Source: CAD feature listing. Evaluate the final solid. Frame: model axes, mm. Coordinates: 2 decimals unless noted, no trailing zeros. Order: outer loops, then holes, each group sorted by start corner. A loop starts at its lowest first (then second) coordinate and runs counter-clockwise, first axis right, second up. Notation, with made-up numbers: (81.25, 55) -> (135.25, 55) arc R21 cw to (135.25, 76) -> close; hole circle Ø5 at (38, 66). An arc over 180 degrees is marked (long way). Write item = value, one per line. Start each with the question number.
Item 1: Ray query, line 1 along X through (y, z) = (5, -38); line 2 along X through (y, z) = (14.25, 42); line 3 along Z through (x, y) = (210.5, 2.75). Return the intervals inside material, ascending. Write a range as [from, to].
Item 2: Contact query for flat-ended pins moving along their axis: pin 1 (1 mm diameter, centred on x = -160.5, z = 70.5, fed in from -Y); pin 2 (5 mm diameter, centred on y = 2.5, z = 75.5, fed in from -X). Output: stop coordinate, or through.
Item 3: Section query A-A (z = 84.5). Output: boundary loops of the cut face in (x, y), then the cut area to 3 significant figures.
```python
from build123d import *

# Parameters (mm, degrees)
BOSS_EXTRUDE1_DEPTH = 15
CUT_EXTRUDE2_DEPTH  = 16
SKETCH4_W           = 524.5681158
SKETCH4_H           = 94.971164408
CUT_EXTRUDE3_DEPTH  = 30


with BuildPart() as part:
    # Sketch1 → Boss-Extrude1 (new body)
    with BuildSketch(Plane(origin=(0, 0, 0), x_dir=(1, 0, 0), z_dir=(0, 1, 0))):
        with BuildLine():
            Line((-200, -100), (200, -100))
            ThreePointArc((200, -100), (221.213203436, -91.213203436), (230, -70))
            Line((230, -70), (230, 100))
            Line((230, 100), (-230, 100))
            Line((-230, 100), (-230, -70))
            ThreePointArc((-230, -70), (-221.213203436, -91.213203436), (-200, -100))
        make_face()
    extrude(amount=BOSS_EXTRUDE1_DEPTH)

    # Sketch3 → Cut-Extrude2 (cut, through all)
    with BuildSketch(Plane(origin=(0, 15, 0), x_dir=(1, 0, 0), z_dir=(0, 1, 0))):
        with BuildLine():
            Line((-2466.524123707, -5837.229065469), (-2474.461623707, -5841.991565469))
            ThreePointArc((-2474.461623707, -5841.991565469), (-2480.995719801, -5840.358041446), (-2479.362195777, -5833.823945352))
            Line((-2479.362195777, -5833.823945352), (-2471.424695777, -5829.061445352))
            ThreePointArc((-2471.424695777, -5829.061445352), (-2464.890599684, -5830.694969376), (-2466.524123707, -5837.229065469))
        make_face()
        with BuildLine():
            Line((-2466.524123707, -5905.261445352), (-2474.461623707, -5900.498945352))
            ThreePointArc((-2474.461623707, -5900.498945352), (-2480.995719801, -5902.132469376), (-2479.362195777, -5908.666565469))
            Line((-2479.362195777, -5908.666565469), (-2471.424695777, -5913.429065469))
            ThreePointArc((-2471.424695777, -5913.429065469), (-2464.890599684, -5911.795541446), (-2466.524123707, -5905.261445352))
        make_face()
        with BuildLine():
            Line((-2395.224695777, -5837.229065469), (-2387.287195777, -5841.991565469))
            ThreePointArc((-2387.287195777, -5841.991565469), (-2380.753099684, -5840.358041446), (-2382.386623707, -5833.823945352))
            Line((-2382.386623707, -5833.823945352), (-2390.324123707, -5829.061445352))
            ThreePointArc((-2390.324123707, -5829.061445352), (-2396.858219801, -5830.694969376), (-2395.224695777, -5837.229065469))
        make_face()
        with BuildLine():
            Line((-2395.224695777, -5905.261445352), (-2387.287195777, -5900.498945352))
            ThreePointArc((-2387.287195777, -5900.498945352), (-2380.753099684, -5902.132469376), (-2382.386623707, -5908.666565469))
            Line((-2382.386623707, -5908.666565469), (-2390.324123707, -5913.429065469))
            ThreePointArc((-2390.324123707, -5913.429065469), (-2396.858219801, -5911.795541446), (-2395.224695777, -5905.261445352))
        make_face()
        with BuildLine():
            Line((-34.016189941, -35.649713965), (-29.253689941, -43.587213965))
            ThreePointArc((-29.253689941, -43.587213965), (-30.887213965, -50.121310059), (-37.421310059, -48.487786035))
            Line((-37.421310059, -48.487786035), (-42.183810059, -40.550286035))
            ThreePointArc((-42.183810059, -40.550286035), (-40.550286035, -34.016189941), (-34.016189941, -35.649713965))
        make_face()
        with BuildLine():
            Line((34.016189941, -35.649713965), (29.253689941, -43.587213965))
            ThreePointArc((29.253689941, -43.587213965), (30.887213965, -50.121310059), (37.421310059, -48.487786035))
            Line((37.421310059, -48.487786035), (42.183810059, -40.550286035))
            ThreePointArc((42.183810059, -40.550286035), (40.550286035, -34.016189941), (34.016189941, -35.649713965))
        make_face()
        with BuildLine():
            Line((-34.016189941, 35.649713965), (-29.253689941, 43.587213965))
            ThreePointArc((-29.253689941, 43.587213965), (-30.887213965, 50.121310059), (-37.421310059, 48.487786035))
            Line((-37.421310059, 48.487786035), (-42.183810059, 40.550286035))
            ThreePointArc((-42.183810059, 40.550286035), (-40.550286035, 34.016189941), (-34.016189941, 35.649713965))
        make_face()
        with BuildLine():
            Line((34.016189941, 35.649713965), (29.253689941, 43.587213965))
            ThreePointArc((29.253689941, 43.587213965), (30.887213965, 50.121310059), (37.421310059, 48.487786035))
            Line((37.421310059, 48.487786035), (42.183810059, 40.550286035))
            ThreePointArc((42.183810059, 40.550286035), (40.550286035, 34.016189941), (34.016189941, 35.649713965))
        make_face()
    extrude(amount=-CUT_EXTRUDE2_DEPTH, mode=Mode.SUBTRACT)

    # Sketch4 → Cut-Extrude3 (cut)
    with BuildSketch(Plane(origin=(0, 0, -100), x_dir=(-1, 0, 0), z_dir=(0, 0, -1))):
        Rectangle(SKETCH4_W, SKETCH4_H)
    extrude(amount=-CUT_EXTRUDE3_DEPTH, mode=Mode.SUBTRACT)


solid = part.part
```
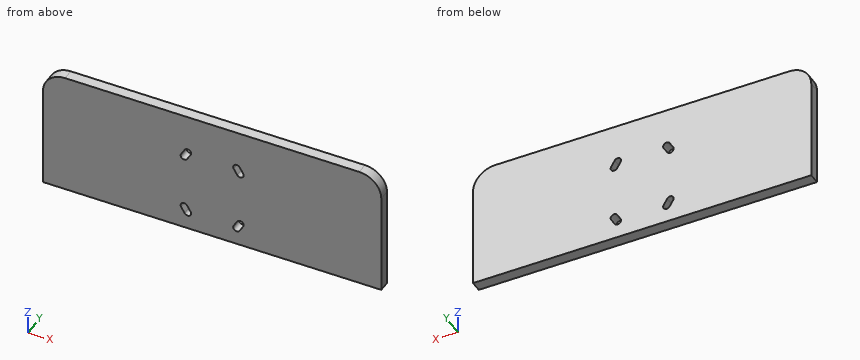
Computed:
q1.line_1 = [-230, -42.86], [-32.61, 32.61], [42.86, 230]
q1.line_2 = [-230, -41.31], [-30.21, 30.21], [41.31, 230]
q1.line_3 = [-70, 98.1]
q2.pin_1 = 0
q2.pin_2 = -229.85
q3.outline = (-226.26, 0) -> (226.26, 0) -> (226.26, 15) -> (-226.26, 15) -> close
q3.area = 6,790 mm^2
